Job drawing, mm, ordinate dimensions from the low corner. One solid piece. A direction names the side the tool comes from. Give positions to 0.01 mm unless a question says otherwise; leave off trailing zeros. Write each loop counter-clockwise with the first axis right and the second up, starting at its lowest first coordinate (ties: lowest second). Pieces come first, ordered by that corner, then holes. Notation, with made-up numbers: (-35, 75.5) - (5, 75.5) arc R9 ccw to (5, 91.5) - close; hole circle Ø7 at (86, 62). An arc over 180 degrees is marked (long way). Answer as a JSON object with one key per item and string values.
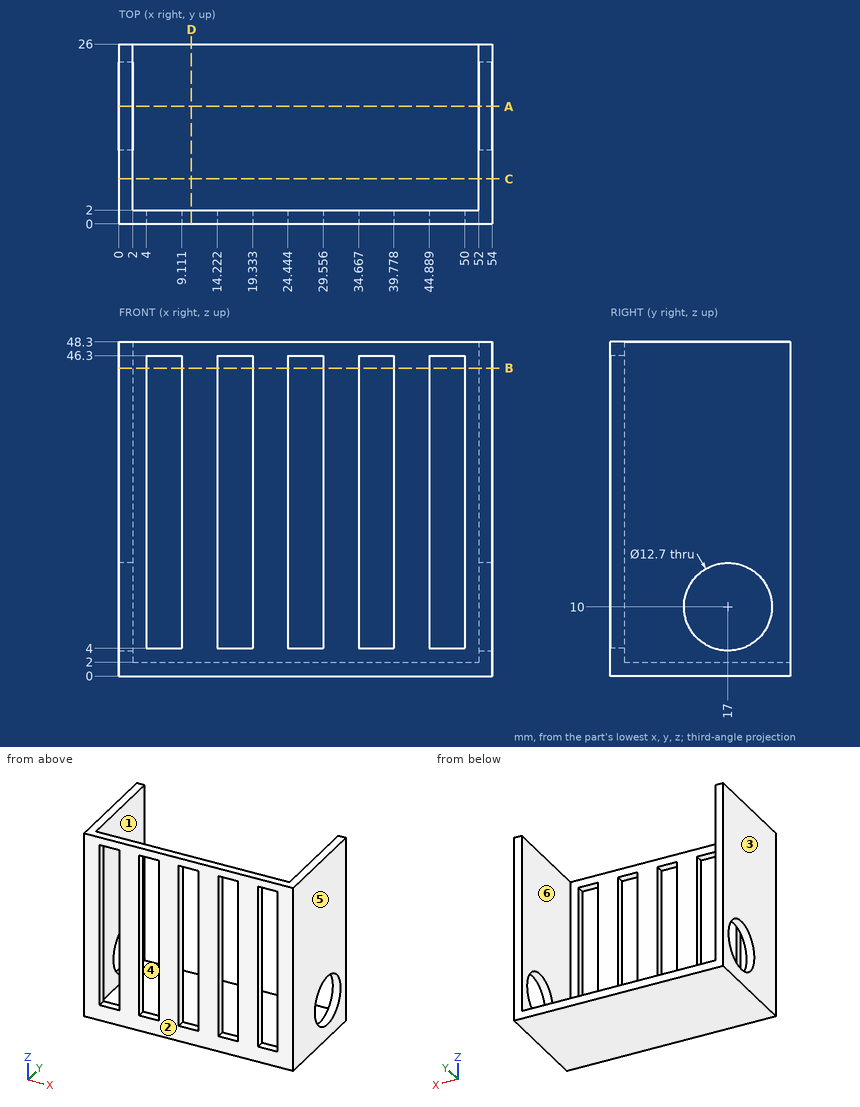
Item 1: Cut at A-A (y = 17). Give the cut face in (x, z).
Entries:
{"outline": "(0, 0) - (54, 0) - (54, 3.65) - (52, 3.65) - (52, 2) - (2, 2) - (2, 3.65) - (0, 3.65) - close; (0, 16.35) - (2, 16.35) - (2, 48.3) - (0, 48.3) - close; (52, 16.35) - (54, 16.35) - (54, 48.3) - (52, 48.3) - close"}
Item 2: Probe line 1 (Z direction, x = 1.4, y = 17); line 2 (Y direction, x = 1.5, z = 10); line 3 (X direction, y = 17, z = 42). List the from-to ranges inside material, lowest first. Write a range as from..to.
Entries:
{"line 1": "0..3.65, 16.35..48.3", "line 2": "0..10.65, 23.35..26", "line 3": "0..2, 52..54"}
Item 3: Cut at D-D (x = 10.5). Give the cut face in (y, z).
Entries:
{"outline": "(0, 0) - (26, 0) - (26, 2) - (2, 2) - (2, 48.3) - (0, 48.3) - close"}
Item 4: Flat gauge pins, fed straight in: P1, Ø1.5, axis at x = 44, z = 15.5, coming from the +Y side; P2, Ø1, axis at x = 41, y = 8.5, coming from the +Z side; P3, Ø11.5, axis at y = 17, z = 10, coming from the -X side. Where does each tip first touch, or does it go through?
Entries:
{"P1": "y = 2", "P2": "z = 2", "P3": "through"}
Item 5: Which spindle directions (+Z, -Z, +X, -X, +Y, -Y) get a long thin tool onto all of the face, cutting with end or side? Do the marked faces 5 and 6. Say none if no direction does.
Entries:
{"face 5": "+Z, -Z, +X, +Y, -Y", "face 6": "+Z, +Y"}
Item 6: Cut at C-C (y = 6.5). Give the cut face in (x, z).
Entries:
{"outline": "(0, 0) - (54, 0) - (54, 48.3) - (52, 48.3) - (52, 2) - (2, 2) - (2, 48.3) - (0, 48.3) - close"}
Item 7: Mould opens along X. For the marked faces 1, 2, 3 and 4 say: +X half, -X half, draft (parallel to the pull), parting line (faces both ways), or undercut.
Entries:
{"face 1": "undercut", "face 2": "draft", "face 3": "-X half", "face 4": "undercut"}
Item 8: Cut at B-B (z = 44.5). Give the cut face in (x, y) (1 decimal), and give its area (3 significant figures).
Entries:
{"outline": "(0, 0) - (4, 0) - (4, 2) - (2, 2) - (2, 26) - (0, 26) - close; (9.1, 0) - (14.2, 0) - (14.2, 2) - (9.1, 2) - close; (19.3, 0) - (24.4, 0) - (24.4, 2) - (19.3, 2) - close; (29.6, 0) - (34.7, 0) - (34.7, 2) - (29.6, 2) - close; (39.8, 0) - (44.9, 0) - (44.9, 2) - (39.8, 2) - close; (50, 0) - (54, 0) - (54, 26) - (52, 26) - (52, 2) - (50, 2) - close", "area": "153 mm2"}
